For this review, take the finished solid that the model builds, in its own axes (mm). A direction names the side the tool comes from. Round coordinates to 2 decimals unless told otherwise and drop trailing zeros. Write each loop counter-clockwise with the first axis right and the second up, starting at its lowest first coordinate (ties: lowest second). Pieces come first, ordered by that corner, then holes. Notation, with made-up numbers: (-18, -3) -> (4, -3) arc R31 cw to (4, 35) -> close; hole circle Ø4 at (-38, 82). An arc over 180 degrees is marked (long way). Answer in a Markdown table with one row per item.
from build123d import *

# Parameters (mm, degrees)
F1_DEPTH = 260.35
F2_R     = 1.190625
F3_DEPTH = 12.701
F4_R     = 1.778
F5_DEPTH = 12.701
F6_W     = 9.525
F6_H     = 9.525
F7_DEPTH = 19.05


with BuildPart() as f1:
    # F0 (on Top) → F1 (new body)
    with BuildSketch(Plane.XY):
        Polygon((-4.7625, -4.7625), (-4.7625, 4.7625), (0, 4.7625), (0, 6.35), (-6.35, 6.35), (-6.35, -6.35), (6.35, -6.35), (6.35, 0), (4.7625, 0), (4.7625, -4.7625), align=None)
        Polygon((0, 6.35), (0, 4.7625), (4.7625, 4.7625), (4.7625, 0), (6.35, 0), (6.35, 6.35), align=None)
        Polygon((0, 4.7625), (-4.7625, 4.7625), (-4.7625, -4.7625), (4.7625, -4.7625), (4.7625, 0), (4.7625, 4.7625), align=None)
    extrude(amount=F1_DEPTH)

    # F2 (on face) → F3 (cut, through all)
    with BuildSketch(Plane.YZ.offset(6.35)):
        with Locations((0, 254)):
            Circle(F2_R)
        with Locations((0, 247.65)):
            Circle(F2_R)
    extrude(amount=-F3_DEPTH, mode=Mode.SUBTRACT)

    # F4 (on face) → F5 (cut, through all)
    with BuildSketch(Plane.YZ.offset(6.35)):
        with BuildLine():
            ThreePointArc((-4.7625, 38.1), (0, 33.3375), (4.7625, 38.1))
            Line((4.7625, 38.1), (-4.7625, 38.1))
        make_face()
        with BuildLine():
            Line((-4.7625, 38.1), (4.7625, 38.1))
            ThreePointArc((4.7625, 38.1), (0, 42.8625), (-4.7625, 38.1))
        make_face()
        with Locations((0, 57.15)):
            Circle(F4_R)
        with Locations((0, 69.85)):
            Circle(F4_R)
        with Locations((0, 19.05)):
            Circle(F4_R)
        with Locations((0, 6.35)):
            Circle(F4_R)
    extrude(amount=-F5_DEPTH, mode=Mode.SUBTRACT)

    # F6 (on face) → F7 (cut)
    with BuildSketch(Plane.XY.offset(260.35)):
        Rectangle(F6_W, F6_H)
    extrude(amount=-F7_DEPTH, mode=Mode.SUBTRACT)


solid = f1.part
1) Consider section A-A on z = 38.1. State the section outline as (x, y) points.
Solved:
| item | result |
|---|---|
| outline | (-6.35, -6.35) -> (6.35, -6.35) -> (6.35, -4.76) -> (-6.35, -4.76) -> close; (-6.35, 4.76) -> (6.35, 4.76) -> (6.35, 6.35) -> (-6.35, 6.35) -> close |
2) For line 1 (X direction, y = 1.5, z = 243); line 2 (Z direction, x = -3.5, y = 0); line 3 (Z direction, x = 4.5, y = 1.25), list the stretches that pass through material, from the lowest coordinate up. Write a range as [from, to].
Solved:
| item | result |
|---|---|
| line 1 | [-6.35, -4.76], [4.76, 6.35] |
| line 2 | [0, 4.57], [8.13, 17.27], [20.83, 33.34], [42.86, 55.37], [58.93, 68.07], [71.63, 241.3] |
| line 3 | [0, 5.09], [7.61, 17.79], [20.31, 33.5], [42.7, 55.89], [58.41, 68.59], [71.11, 241.3] |
3) Clearance check with flat-ended pins moving along their axes: pin 1 Ø4 at (y, z) = (0, 254) entering from -X; pin 2 Ø4 at (x, y) = (-2.5, -1) entering from +Z. State where each tip first meets the part, or that it passes through.
Solved:
| item | result |
|---|---|
| pin 1 | x = -6.35 |
| pin 2 | z = 241.3 |
4) Mouldability with a two-part tool opening along X and no side actions: class faces 3 (the flat face through (4.762, 0, 251)), 4 (the flat face through (0, 6.35, 128)), 5 (the flat face through (0, 4.762, 251)), 6 (the flat face through (-6.35, 0, 128)) as pulls with the +X half, pulls with the -X half, needs draft (parallel to the pull), parting line crosses it, or undercut.
Solved:
| item | result |
|---|---|
| face 3 | undercut |
| face 4 | needs draft |
| face 5 | undercut |
| face 6 | pulls with the -X half |
5) For faces 1 (the flat face through (-4.762, 0, 251)), 2 (the flat face through (0, 0, 0)), list the 3-axis set-ups (+Z, -Z, +X, -X, +Y, -Y) from which the entire face can be reached by the end or side of a thin tool; tool diameter is ignored.
Solved:
| item | result |
|---|---|
| face 1 | +Z |
| face 2 | -Z, +X, -X, +Y, -Y |
6) Consider section B-B on x = 0.5. State how many separate pieces and enclosed holes the cut face has, then the cut area to 3 significant figures.
Solved:
| item | result |
|---|---|
| separate pieces | 1 |
| enclosed holes | 5 |
| area | 3,010 mm² |
